Build history of the part. All positions in model axes, mm. Face numbers are marked on the shaded views. Round coordinates to 2 decimals unless told otherwise and drop trailing zeros. Write each loop counter-clockwise with the first axis right and the second up, starting at its lowest first coordinate (ties: lowest second). Pieces come first, ordered by that corner, then holes. Notation, with made-up numbers: (-33.5, -39) -> (-17.5, -39) arc R9 ccw to (-17.5, -35) -> close; hole circle Ø4 at (-14, 5). An arc over 180 degrees is marked (long way). One line per question, with ' | ' between items.
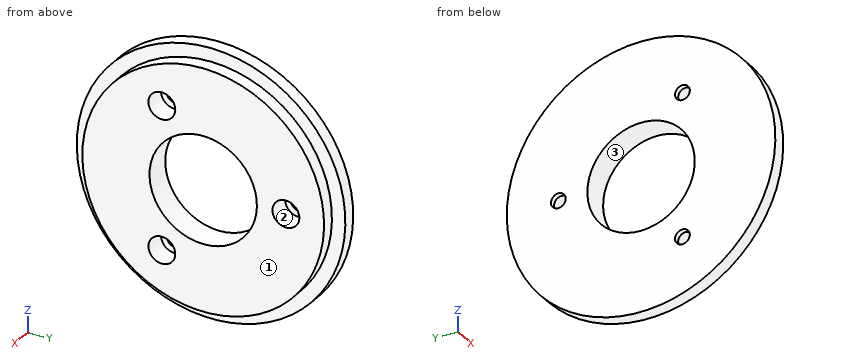
from build123d import *

# Parameters (mm, degrees)
SKETCH4_R          = 3.4925
SKETCH4_R_2        = 25.4
CUT_EXTRUDE1_DEPTH = 91.696141042
SKETCH4_3_R        = 6.35
CUT_EXTRUDE2_DEPTH = 10.16


with BuildPart() as part:
    # Sketch1 → Revolve1 (revolve)
    with BuildSketch(Plane.XY, mode=Mode.PRIVATE) as revolve1_sk:
        Polygon((0, 0), (0, 57.15), (-6.35, 57.15), (-6.35, 63.5), (-12.7, 63.5), (-12.7, 0), align=None)
    revolve(revolve1_sk.sketch.rotate(Axis((0, 0, 0), (1, 0, 0)), 90), axis=Axis((0, 0, 0), (1, 0, 0)))

    # Sketch4 → Cut-Extrude1 (cut, through all)
    with BuildSketch(Plane(origin=(0, 0, 0), x_dir=(0, 0, -1), z_dir=(1, 0, 0))):
        with Locations((0, 39.116)):
            Circle(SKETCH4_R)
        with Locations((33.875449694, -19.558)):
            Circle(SKETCH4_R)
        with Locations((-33.875449694, -19.558)):
            Circle(SKETCH4_R)
        Circle(SKETCH4_R_2)
    extrude(amount=-CUT_EXTRUDE1_DEPTH, mode=Mode.SUBTRACT)

    # Sketch4_3 → Cut-Extrude2 (cut)
    with BuildSketch(Plane(origin=(0, 0, 0), x_dir=(0, 0, -1), z_dir=(1, 0, 0))):
        with Locations((0, 39.116)):
            Circle(SKETCH4_3_R)
        with Locations((33.875449694, -19.558)):
            Circle(SKETCH4_3_R)
        with Locations((-33.875449694, -19.558)):
            Circle(SKETCH4_3_R)
    extrude(amount=-CUT_EXTRUDE2_DEPTH, mode=Mode.SUBTRACT)


solid = part.part
(1) Wall check: line 1 (Y direction, x = -11.3, z = 0); line 2 (Y direction, x = -7.25, z = 0); line 3 (Z direction, x = -8, y = -23). Give the ranges that are in metal, low to high. Write a range as from..to.
Calculated:
line 1: -63.5..-25.4, 25.4..35.62, 42.61..63.5 | line 2: -63.5..-25.4, 25.4..32.77, 45.47..63.5 | line 3: -59.19..-39.21, -28.54..-10.78, 10.78..28.54, 39.21..59.19
(2) Slice it at C-C (z = 18). Write the cut outline in (x, y), then the cut area to 3 significant figures.
Calculated:
outline: (-12.7, -60.9) -> (-6.35, -60.9) -> (-6.35, -54.24) -> (0, -54.24) -> (0, -17.92) -> (-12.7, -17.92) -> close; (-12.7, 17.92) -> (0, 17.92) -> (0, 54.24) -> (-6.35, 54.24) -> (-6.35, 60.9) -> (-12.7, 60.9) -> close | area: 1,010 mm2
(3) Mould opens along Z. For the marked faces 1, 2 and 3 say: pulls with the +Z half, pulls with the -Z half, needs draft (parallel to the pull), parting line crosses it, or undercut.
Calculated:
face 1: needs draft | face 2: undercut | face 3: undercut
(4) Slice it at B-B (y = 9.5). Write the cut outline in (x, z).
Calculated:
outline: (-12.7, -62.79) -> (-6.35, -62.79) -> (-6.35, -56.35) -> (0, -56.35) -> (0, -23.56) -> (-12.7, -23.56) -> close; (-12.7, 23.56) -> (0, 23.56) -> (0, 56.35) -> (-6.35, 56.35) -> (-6.35, 62.79) -> (-12.7, 62.79) -> close
(5) Drop flat-ended pins along their axis: pin 1 (3 mm diameter, centred on y = -21.5, z = -9, fed in from +X); pin 2 (2 mm diameter, centred on x = -1.5, y = 25.5, fed in from -Z); pin 3 (7.5 mm diameter, centred on y = -19.56, z = 33.88, fed in from +X); pin 4 (4 mm diameter, centred on x = -10, z = 14, fed in from +Y). Give the stop position or say it passes through.
Calculated:
pin 1: through | pin 2: z = -51.63 | pin 3: x = -10.16 | pin 4: y = 62.36
(6) Slice it at A-A (z = 0). Write the cut outline in (x, y).
Calculated:
outline: (-12.7, -63.5) -> (-6.35, -63.5) -> (-6.35, -57.15) -> (0, -57.15) -> (0, -25.4) -> (-12.7, -25.4) -> close; (-12.7, 25.4) -> (0, 25.4) -> (0, 32.77) -> (-10.16, 32.77) -> (-10.16, 35.62) -> (-12.7, 35.62) -> close; (-12.7, 42.61) -> (-10.16, 42.61) -> (-10.16, 45.47) -> (0, 45.47) -> (0, 57.15) -> (-6.35, 57.15) -> (-6.35, 63.5) -> (-12.7, 63.5) -> close
(7) Slice it at D-D (y = 28). Write the cut outline in (x, z), then the cut area to 3 significant figures.
Calculated:
outline: (-12.7, -56.99) -> (-6.35, -56.99) -> (-6.35, -49.82) -> (0, -49.82) -> (0, 49.82) -> (-6.35, 49.82) -> (-6.35, 56.99) -> (-12.7, 56.99) -> close | area: 1,360 mm2
